```python
from build123d import *

# Parameters (mm, degrees)
SKETCH1_R           = 10
BOSS_EXTRUDE1_DEPTH = 10.5
SKETCH3_R           = 17
BOSS_EXTRUDE2_DEPTH = 12
SKETCH4_R           = 1.55
CUT_EXTRUDE3_DEPTH  = 33.927951652
SKETCH5_R           = 1.55
CUT_EXTRUDE5_DEPTH  = 33.927951652
SKETCH6_R           = 1.75
CUT_EXTRUDE6_DEPTH  = 5.2
SKETCH7_R           = 1.75
CUT_EXTRUDE7_DEPTH  = 18.5
SKETCH8_R           = 6.5
CUT_EXTRUDE8_DEPTH  = 13.5


with BuildPart() as part:
    # Sketch1 → Boss-Extrude1 (new body)
    with BuildSketch(Plane.XY):
        with Locations(Location((0, 0, 0), (0, 0, 180))):
            Circle(SKETCH1_R)
    extrude(amount=BOSS_EXTRUDE1_DEPTH)

    # Sketch3 → Boss-Extrude2 (add)
    with BuildSketch(Plane.XY.offset(10.5)):
        Circle(SKETCH3_R)
    extrude(amount=BOSS_EXTRUDE2_DEPTH)

    # Sketch4 → Cut-Extrude3 (cut, through all)
    with BuildSketch(Plane.XY.offset(22.5)):
        with Locations((3, 0)):
            Circle(SKETCH4_R)
        with Locations((-3, 0)):
            Circle(SKETCH4_R)
    extrude(amount=-CUT_EXTRUDE3_DEPTH, mode=Mode.SUBTRACT)

    # Sketch5 → Cut-Extrude5 (cut, through all)
    with BuildSketch(Plane.XY.offset(22.5)):
        with Locations((13, 0)):
            Circle(SKETCH5_R)
        with Locations((0, -13)):
            Circle(SKETCH5_R)
        with Locations((-13, 0)):
            Circle(SKETCH5_R)
        with Locations((0, 13)):
            Circle(SKETCH5_R)
    extrude(amount=-CUT_EXTRUDE5_DEPTH, mode=Mode.SUBTRACT)

    # Sketch6 → Cut-Extrude6 (cut)
    with BuildSketch(Plane(origin=(0, 0, 10.5), x_dir=(-1, 0, 0), z_dir=(0, 0, -1))):
        with Locations((13, 0)):
            Circle(SKETCH6_R)
        with Locations((0, -13)):
            Circle(SKETCH6_R)
        with Locations((-13, 0)):
            Circle(SKETCH6_R)
        with Locations((0, 13)):
            Circle(SKETCH6_R)
    extrude(amount=-CUT_EXTRUDE6_DEPTH, mode=Mode.SUBTRACT)

    # Sketch7 → Cut-Extrude7 (cut)
    with BuildSketch(Plane.XY.offset(22.5)):
        with Locations((3, 0)):
            Circle(SKETCH7_R)
        with Locations((-3, 0)):
            Circle(SKETCH7_R)
    extrude(amount=-CUT_EXTRUDE7_DEPTH, mode=Mode.SUBTRACT)

    # Sketch8 → Cut-Extrude8 (cut)
    with BuildSketch(Plane.XY.offset(22.5)):
        Circle(SKETCH8_R)
    extrude(amount=-CUT_EXTRUDE8_DEPTH, mode=Mode.SUBTRACT)


solid = part.part
```
Design review of the part built by this model. Coordinates are the model's own, in mm. A direction names the side the tool comes from. Coordinates: 2 decimals unless noted, no trailing zeros. Order: outer loops, then holes, each group sorted by start corner. A loop starts at its lowest first (then second) coordinate and runs counter-clockwise, first axis right, second up. Notation, with made-up numbers: M -22.5,57 L 21.5,57 A10 cw 21.5,75 Z; hole C -5,-40 d6. An arc over 180 degrees is marked long. Answer as a JSON object with one key per item and string values. Group by question number.
1) Add section B-B, the plane x = -12. Write out the cut boundary in (y, z).
2) Wall thickness on L1, parallel to Y at x = -0.5, z = 13.25; L2, parallel to Z at x = -15, y = 5; L3, parallel to Z at x = -3, y = 5: over which ranges is each line inside the solid? List them lowest first.
3) For pin 1 (6 mm diameter, centred on x = 12, z = 14, fed in from -Y); pin 2 (1 mm diameter, centred on y = 13.5, z = 13, fed in from +X); pin 3 (4.5 mm diameter, centred on x = 0, y = 13, fed in from -Z), all flat-tipped, find the tip position at first contact; note any pin that passes through.
4) Tool access review of faces 1 (the cylindrical face through (9.139, 14.334, 16.416)), 2 (the cylindrical face through (11.331, 0.526, 13.064)): name each direction out of +Z, -Z, +X, -X, +Y, -Y from which nothing blocks a thin tool from reaching the whole face with its end or side.
5) Mouldability with a two-part tool opening along X and no side actions: class faces 3 (the flat face through (7.3, -7.3, 10.5)), 4 (the cylindrical face through (-5.158, -3.955, 15.844)), 5 (the cylindrical face through (10, 0, 5)) as pulls with the +X half, pulls with the -X half, needs draft (parallel to the pull), parting line crosses it, or undercut.
6) Add section A-A, the plane z = 18.75. Write out the cut boundary in (x, y).
7) Add section C-C, the plane y = -13. Write out the cut boundary in (x, z), then the cut area to 3 significant figures.
8) Add section D-D, the plane y = 0. Count the separate pieces of the cut face and the enclosed holes in it, then the cut area to 3 significant figures.
Computed values:
{
 "1": {"outline": "M -12.04,10.5 L -1.44,10.5 L -1.44,15.7 L -1.18,15.7 L -1.18,22.5 L -12.04,22.5 Z; M 1.18,15.7 L 1.44,15.7 L 1.44,10.5 L 12.04,10.5 L 12.04,22.5 L 1.18,22.5 Z"},
 "2": {"L1": "y = -16.99 to -14.68, -11.32 to -6.48, 6.48 to 11.32, 14.68 to 16.99", "L2": "z = 10.5 to 22.5", "L3": "z = 0 to 9"},
 "3": {"pin 1": "stops at y = -14.42", "pin 2": "stops at x = 10.95", "pin 3": "stops at z = 10.5"},
 "4": {"face 1": "+Z, -Z", "face 2": "-Z"},
 "5": {"face 3": "needs draft", "face 4": "undercut", "face 5": "parting line crosses it"},
 "6": {"outline": "C 0,0 d34; hole C -13,0 d3.1; hole C 0,0 d13; hole C 0,-13 d3.1; hole C 0,13 d3.1; hole C 13,0 d3.1"},
 "7": {"outline": "M -10.95,10.5 L -1.75,10.5 L -1.75,15.7 L -1.55,15.7 L -1.55,22.5 L -10.95,22.5 Z; M 1.55,15.7 L 1.75,15.7 L 1.75,10.5 L 10.95,10.5 L 10.95,22.5 L 1.55,22.5 Z", "area": "224 mm^2"},
 "8": {"separate pieces": "5", "enclosed holes": "0", "area": "304 mm^2"}
}
